Part print with two shaded views. Sizes in mm from the minimum x, y, z corner. A direction names the side the tool comes from. Round coordinates to 2 decimals unless told otherwise and drop trailing zeros. Write each loop counter-clockwise with the first axis right and the second up, starting at its lowest first coordinate (ties: lowest second). Pieces come first, ordered by that corner, then holes. Notation, with made-up numbers: (31.5, 63.25) - (61.5, 63.25) arc R15 ccw to (61.5, 77.25) - close; hole circle Ø9 at (55.25, -17). An arc over 180 degrees is marked (long way). Answer as a JSON object with one key per item and string values. Group by question number.
Item 1: Flat gauge pins, fed straight in: pin 1 (1 mm diameter, centred on y = 248.5, z = 244, fed in from +X); pin 2 (4 mm diameter, centred on y = 381.5, z = 637, fed in from -X); pin 3 (6 mm diameter, centred on x = 491.5, y = 134, fed in from +Z). Where does each tip first touch, or does it go through?
Item 2: Slice it at D-D, the plane x = 760. List the corners of the cut face in (y, z).
Item 3: Slice it at A-A, the plane z = 406.4. List the corners of the cut face in (x, y), then the cut area to 3 significant figures.
Item 4: Slice it at B-B, the plane x = 406.4. List the corners of the cut face in (y, z).
Item 5: Which spindle directions (+Z, -Z, +X, -X, +Y, -Y) get a long thin tool onto all of the face, cutting with end or side? Do the marked faces 1 and 2. Say none if no direction does.
Item 6: Slice it at C-C, the plane y = 150. List the corners of the cut face in (x, z).
Item 7: Probe line 1 (Z direction, x = 406.4, y = 497.5); line 2 (X direction, y = 280, z = 406). List the from-to ranges inside material, lowest first. Write a range as from..to.
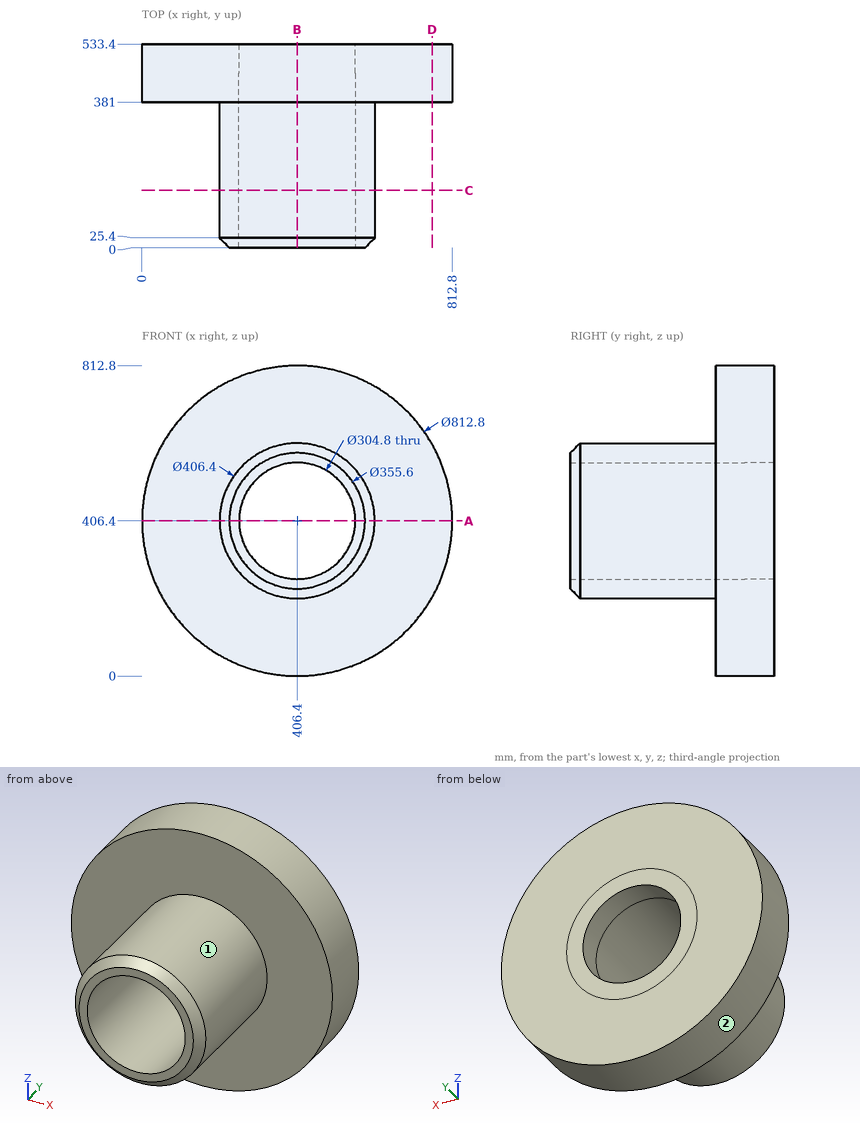
Geometry says:
{
 "1": {"pin 1": "stops at x = 529.2", "pin 2": "stops at x = 70.39", "pin 3": "stops at z = 592.28"},
 "2": {"outline": "(381, 206.08) - (533.4, 206.08) - (533.4, 606.72) - (381, 606.72) - close"},
 "3": {"outline": "(0, 381) - (203.2, 381) - (203.2, 25.4) - (228.6, 0) - (254, 0) - (254, 533.4) - (0, 533.4) - close; (558.8, 0) - (584.2, 0) - (609.6, 25.4) - (609.6, 381) - (812.8, 381) - (812.8, 533.4) - (558.8, 533.4) - close", "area": "115,000 mm^2"},
 "4": {"outline": "(0, 228.6) - (25.4, 203.2) - (381, 203.2) - (381, 0) - (533.4, 0) - (533.4, 254) - (0, 254) - close; (0, 558.8) - (533.4, 558.8) - (533.4, 812.8) - (381, 812.8) - (381, 609.6) - (25.4, 609.6) - (0, 584.2) - close"},
 "5": {"face 1": "-Y", "face 2": "+Y, -Y"},
 "6": {"outline": "circle Ø406.4 at (406.4, 406.4); hole circle Ø304.8 at (406.4, 406.4)"},
 "7": {"line 1": "z = 0..254, 558.8..812.8", "line 2": "x = 203.2..254, 558.8..609.6"}
}
